Drawing for the job (mm, zero at the part's lowest x, y, z). A direction names the side the tool comes from. Give positions to 0.01 mm unless a question says otherwise; leave off trailing zeros. Order: outer loops, then holes, each group sorted by start corner. A loop starts at its lowest first (then second) coordinate and runs counter-clockwise, first axis right, second up. Notation, with made-up numbers: (6.5, 43) -> (47.5, 43) arc R14 ccw to (47.5, 64) -> close; hole circle Ø8 at (-32, -39). An arc over 180 degrees is marked (long way). Use a Markdown table: item, result. Add a question column.
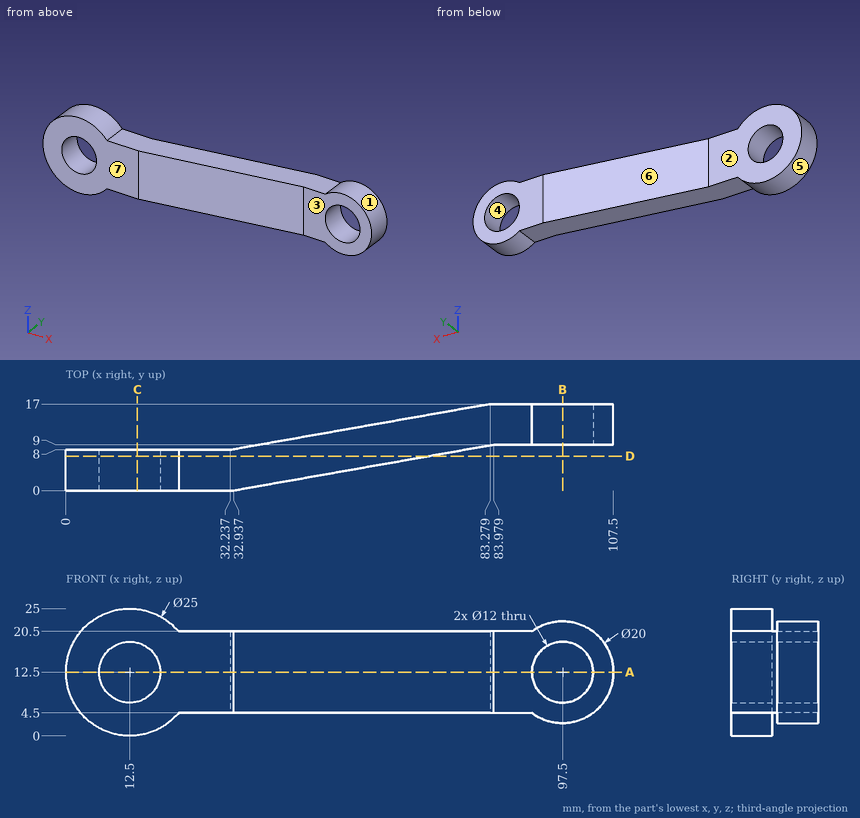
(1) Band-saw the part on B-B on x = 97.5. Give the cut face in (y, z).
(2) Band-saw the part on D-D on y = 6.75. Give the cut face in (x, z) (1 decimal).
(3) Band-saw the part on C-C on x = 14. Give the cut face in (y, z).
(4) Pin check, flat tips, straight feed: pin 1 Ø2 at (y, z) = (14.5, 18.5) entering from +X; pin 2 Ø8 at (y, z) = (4.5, 22) entering from -X (1 decimal); pin 3 Ø10 at (x, z) = (59.5, 15.5) entering from -Y. Stop position of each tip, or through.
(5) Mould opens along X. For the marked faces 4, 5, 6 and 7 say: released by +X, released by -X, zero draft, split by the parting line, or undercut.
(6) Tool access for the marked faces 1, 2 and 3: list every direction of +Z, -Z, +X, -X, +Y, -Y with a clear straight run to the whole face (end or side of a thin tool).
(7) Band-saw the part on A-A on z = 12.5. Give the cut face in (x, y).
(8) Wall check: probe 1 along Z at (x, y) = (97.5, 13); probe 2 along Z at (x, y) = (12.5, 3.25); probe 3 along Z at (x, y) = (66.5, 9.75). Give the ranges that are in metal, low to high.
Response:
| question | item | result |
|---|---|---|
| 1 | outline | (9, 2.5) -> (17, 2.5) -> (17, 6.5) -> (9, 6.5) -> close; (9, 18.5) -> (17, 18.5) -> (17, 22.5) -> (9, 22.5) -> close |
| 2 | outline | (22.1, 4.5) -> (71.2, 4.5) -> (71.2, 20.5) -> (22.1, 20.5) arc R12.5 ccw (long way) to start; hole circle Ø12 at (12.5, 12.5) |
| 3 | outline | (0, 0.09) -> (8, 0.09) -> (8, 6.69) -> (0, 6.69) -> close; (0, 18.31) -> (8, 18.31) -> (8, 24.91) -> (0, 24.91) -> close |
| 4 | pin 1 | stops at x = 106.16 |
| 4 | pin 2 | stops at x = 1.3 |
| 4 | pin 3 | stops at y = 3.8 |
| 5 | face 4 | undercut |
| 5 | face 5 | split by the parting line |
| 5 | face 6 | released by -X |
| 5 | face 7 | zero draft |
| 6 | face 1 | +Y, -Y |
| 6 | face 2 | +Z, -Z, -X, +Y |
| 6 | face 3 | +Z, -Z, +X, -Y |
| 7 | outline | (0, 0) -> (6.5, 0) -> (6.5, 8) -> (0, 8) -> close; (18.5, 0) -> (32.94, 0) -> (83.98, 9) -> (91.5, 9) -> (91.5, 17) -> (83.28, 17) -> (32.24, 8) -> (18.5, 8) -> close; (103.5, 9) -> (107.5, 9) -> (107.5, 17) -> (103.5, 17) -> close |
| 8 | probe 1 | z = 2.5 to 6.5, 18.5 to 22.5 |
| 8 | probe 2 | z = 0 to 6.5, 18.5 to 25 |
| 8 | probe 3 | z = 4.5 to 20.5 |
